Geometry check sheet. Reference: the model listing, model coordinates, mm. Coordinates: 2 decimals unless noted, no trailing zeros. Write each loop counter-clockwise with the first axis right and the second up, starting at its lowest first coordinate (ties: lowest second). Pieces come first, ordered by that corner, then holes. Notation, with made-up numbers: (59.25, 11) -> (92.25, 11) arc R25 cw to (92.25, 49) -> close; hole circle Ø3 at (-36.75, 65). An arc over 180 degrees is marked (long way). Use a Markdown table: item, result.
```python
from build123d import *

# Parameters (mm, degrees)
F0_R     = 11.5
F1_DEPTH = 2.4


with BuildPart() as f1:
    # F0 (on Front) → F1 (new body)
    with BuildSketch(Plane.XZ):
        with BuildLine():
            Line((15.31951195, 19.8149923235), (-15.31951195, 19.8149923235))
            ThreePointArc((-15.31951195, 19.8149923235), (-18.1479390748, 18.6434194483), (-19.31951195, 15.8149923235))
            Line((-19.31951195, 15.8149923235), (-19.31951195, -15.8149923235))
            ThreePointArc((-19.31951195, -15.8149923235), (-18.1479390748, -18.6434194483), (-15.31951195, -19.8149923235))
            Line((-15.31951195, -19.8149923235), (15.31951195, -19.8149923235))
            ThreePointArc((15.31951195, -19.8149923235), (18.1479390748, -18.6434194483), (19.31951195, -15.8149923235))
            Line((19.31951195, -15.8149923235), (19.31951195, 15.8149923235))
            ThreePointArc((19.31951195, 15.8149923235), (18.1479390748, 18.6434194483), (15.31951195, 19.8149923235))
        make_face()
        with BuildLine():
            ThreePointArc((-17.5, 15.5), (-16.9142135624, 16.9142135624), (-15.5, 17.5))
            Line((-15.5, 17.5), (15.5, 17.5))
            ThreePointArc((15.5, 17.5), (16.9142135624, 16.9142135624), (17.5, 15.5))
            Line((17.5, 15.5), (17.5, -15.5))
            ThreePointArc((17.5, -15.5), (16.9142135624, -16.9142135624), (15.5, -17.5))
            Line((15.5, -17.5), (-15.5, -17.5))
            ThreePointArc((-15.5, -17.5), (-16.9142135624, -16.9142135624), (-17.5, -15.5))
            Line((-17.5, -15.5), (-17.5, 15.5))
        make_face(mode=Mode.SUBTRACT)
        with BuildLine():
            ThreePointArc((-15.5, 17.5), (-14.0857864376, 16.9142135624), (-13.5, 15.5))
            ThreePointArc((-13.5, 15.5), (-15.5, 13.5), (-17.5, 15.5))
            Line((-17.5, 15.5), (-17.5, -15.5))
            ThreePointArc((-17.5, -15.5), (-15.5, -13.5), (-13.5, -15.5))
            ThreePointArc((-13.5, -15.5), (-14.0857864376, -16.9142135624), (-15.5, -17.5))
            Line((-15.5, -17.5), (15.5, -17.5))
            ThreePointArc((15.5, -17.5), (14.0857864376, -14.0857864376), (17.5, -15.5))
            Line((17.5, -15.5), (17.5, 15.5))
            ThreePointArc((17.5, 15.5), (14.0857864376, 14.0857864376), (15.5, 17.5))
            Line((15.5, 17.5), (-15.5, 17.5))
        make_face()
        Circle(F0_R, mode=Mode.SUBTRACT)
    extrude(amount=F1_DEPTH)


solid = f1.part
```
Item 1: Section check B-B on x = 0. Record the boundary of the cut face in (y, z) (3 decimals).
Answer block:
| item | result |
|---|---|
| outline | (-2.4, -19.815) -> (0, -19.815) -> (0, -11.5) -> (-2.4, -11.5) -> close; (-2.4, 11.5) -> (0, 11.5) -> (0, 19.815) -> (-2.4, 19.815) -> close |
Item 2: Section check D-D on z = -16.5. Record the boundary of the cut face in (x, y), then the cut area to 3 significant figures.
Answer block:
| item | result |
|---|---|
| outline | (-19.26, -2.4) -> (-17.23, -2.4) -> (-17.23, 0) -> (-19.26, 0) -> close; (-13.77, -2.4) -> (13.77, -2.4) -> (13.77, 0) -> (-13.77, 0) -> close; (17.23, -2.4) -> (19.26, -2.4) -> (19.26, 0) -> (17.23, 0) -> close |
| area | 75.8 mm^2 |
Item 3: Thickness scan on L1, parallel to Z at x = 15.5, y = -0.9; L2, parallel to X at y = -1.35, z = 15.5; L3, parallel to Z at x = 0, y = -1.55 (3 decimals). Record the ranges inside material, lowest first. Write a range as [from, to].
Answer block:
| item | result |
|---|---|
| L1 | z = [-19.81, -17.5], [-13.5, 13.5], [17.5, 19.81] |
| L2 | x = [-19.32, -17.5], [-13.5, 13.5], [17.5, 19.32] |
| L3 | z = [-19.815, -11.5], [11.5, 19.815] |
Item 4: Section check A-A on y = -1.95. Record the boundary of the cut face in (x, z) (3 decimals).
Answer block:
| item | result |
|---|---|
| outline | (-19.32, -15.815) arc R4 ccw to (-15.32, -19.815) -> (15.32, -19.815) arc R4 ccw to (19.32, -15.815) -> (19.32, 15.815) arc R4 ccw to (15.32, 19.815) -> (-15.32, 19.815) arc R4 ccw to (-19.32, 15.815) -> close; hole circle Ø4 at (-15.5, -15.5); hole circle Ø4 at (-15.5, 15.5); hole circle Ø23 at (0, 0); hole circle Ø4 at (15.5, -15.5); hole circle Ø4 at (15.5, 15.5) |
Item 5: Mould release check, pull along Z, two halves, no side actions. Record for faces 1 (the flat face through (-19.32, -1, 0)), 2 (the cylindrical face through (18.18, -1.18, 18.61)), 3 (the cylindrical face through (18.12, -1.18, -18.67)), 4 (the cylindrical face through (-1.5, -1.2, 11.4)): +Z half, -Z half, draft (parallel to the pull), parting line (faces both ways), or undercut.
Answer block:
| item | result |
|---|---|
| face 1 | draft |
| face 2 | +Z half |
| face 3 | -Z half |
| face 4 | undercut |
Item 6: Depth check by flat-ended pin: P1, Ø4.5, axis at x = 15.5, z = 15.5, coming from the +Y side; P2, Ø3, axis at x = 15.5, z = -15.5, coming from the +Y side. Enter the tip coordinate at first touch or a pass-through.
Answer block:
| item | result |
|---|---|
| P1 | stops at y = 0 |
| P2 | passes through |
Item 7: Section check C-C on z = 4. Record the boundary of the cut face in (x, y).
Answer block:
| item | result |
|---|---|
| outline | (-19.32, -2.4) -> (-10.78, -2.4) -> (-10.78, 0) -> (-19.32, 0) -> close; (10.78, -2.4) -> (19.32, -2.4) -> (19.32, 0) -> (10.78, 0) -> close |
